Geometry: final body of the model. Coordinates: model frame, mm. Face numbers are marked on the shaded views. A direction names the side the tool comes from. Coordinates: 2 decimals unless noted, no trailing zeros. Write each loop counter-clockwise with the first axis right and the second up, starting at its lowest first coordinate (ties: lowest second). Pieces come first, ordered by that corner, then holes. Notation, with made-up numbers: M -11.75,-34 L 18.25,-34 A22 ccw 18.25,-6 Z; hole C 45.5,-10.5 d6. An arc over 180 degrees is marked long. Write item = value, one per line. Start each with the question number.
Item 1: Reachability of the marked faces 1 and 2 from +Z, -Z, +X, -X, +Y, -Y: full face, straight path, thin tool, end or side. Return the list, or none.
Item 2: First-contact query: pin 1 Ø1 at (x, y) = (10.5, -0.5) entering from -Z. Flat tip, straight axial feed; report the tip coordinate or a pass-through.
Item 3: Ray query, L1, parallel to X at y = 0.5, z = 0; L2, parallel to Y at x = -6, z = 11.5; L3, parallel to Z at x = 0.5, y = -1. Return the intervals inside material, ascending. Write a range as [from, to].
Item 4: Section D-D on y = 2.25. Output: boundary loops of the cut face in (x, z).
Item 5: Pull-direction query (Z, two-part tool) for the marked faces 3 and 4; classes: +Z half, -Z half, draft (parallel to the pull), parting line (faces both ways), or undercut.
Item 6: Section C-C on y = 7. Output: boundary loops of the cut face in (x, z), plus the area to 3 significant figures.
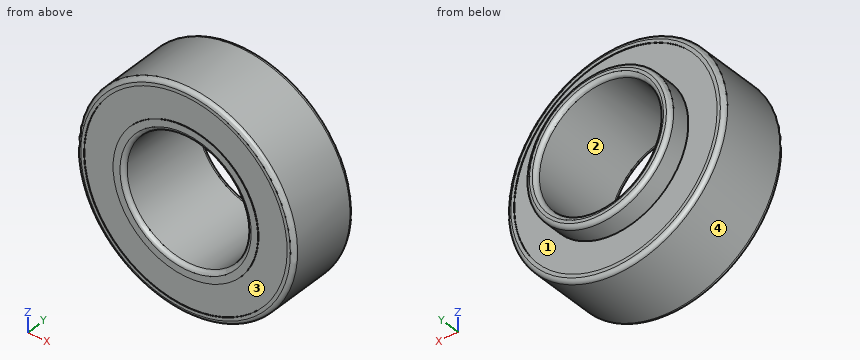
from build123d import *

# Parameters (mm, degrees)
SKETCH1_R           = 15
SKETCH1_R_2         = 8.5
BOSS_EXTRUDE1_DEPTH = 5
SKETCH2_R           = 10
SKETCH2_R_2         = 8.5
BOSS_EXTRUDE2_DEPTH = 3
CUT_EXTRUDE1_START  = -0.05
SKETCH3_R           = 14
SKETCH3_R_2         = 10
CUT_EXTRUDE1_DEPTH  = 0.05
FILLET1_R           = 0.55


with BuildPart() as part:
    # Sketch1 → Boss-Extrude1 (new, symmetric)
    with BuildSketch(Plane(origin=(0, 0, 0), x_dir=(1, 0, 0), z_dir=(0, 1, 0))):
        with Locations(Location((0, 0, 0), (0, 0, 270))):
            Circle(SKETCH1_R)
        with Locations(Location((0, 0, 0), (0, 0, 270))):
            Circle(SKETCH1_R_2, mode=Mode.SUBTRACT)
    extrude(amount=BOSS_EXTRUDE1_DEPTH, both=True)

    # Sketch2 → Boss-Extrude2 (add)
    with BuildSketch(Plane(origin=(0, 5, 0), x_dir=(1, 0, 0), z_dir=(0, 1, 0))):
        with Locations(Location((0, 0, 0), (0, 0, 270))):
            Circle(SKETCH2_R)
        with Locations(Location((0, 0, 0), (0, 0, 270))):
            Circle(SKETCH2_R_2, mode=Mode.SUBTRACT)
    extrude(amount=BOSS_EXTRUDE2_DEPTH)

    # Sketch3 → Cut-Extrude1 (cut)
    with BuildSketch(Plane(origin=(0, 5, 0), x_dir=(1, 0, 0), z_dir=(0, 1, 0)).offset(CUT_EXTRUDE1_START)):
        with Locations(Location((0, 0, 0), (0, 0, 270))):
            Circle(SKETCH3_R)
        with Locations(Location((0, 0, 0), (0, 0, 270))):
            Circle(SKETCH3_R_2, mode=Mode.SUBTRACT)
    cut_extrude1 = extrude(amount=CUT_EXTRUDE1_DEPTH, mode=Mode.SUBTRACT)

    # Mirror1: Cut-Extrude1 across plane
    add(cut_extrude1.mirror(Plane.ZX), mode=Mode.SUBTRACT)

    # Fillet1
    fillet1_edges = [part.edges().sort_by_distance(p)[0] for p in [
        (0, 8, -10),
        (0, 8, -8.5),
        (0, -5, -15),
        (0, 5, -15),
        (0, -5, -8.5),
    ]]
    fillet(fillet1_edges, radius=FILLET1_R)


solid = part.part
Responses:
q1.face_1 = +Y
q1.face_2 = +Y, -Y
q2.pin_1 = -11.18
q3.L1 = [-15, -8.5], [8.5, 15]
q3.L2 = [-4.95, 4.95]
q3.L3 = [-14.99, -8.49], [8.49, 14.99]
q4.outline = C 0,0 d30; hole C 0,0 d17
q5.face_3 = undercut
q5.face_4 = parting line
q6.outline = C 0,0 d20; hole C 0,0 d17
q6.area = 87.2 mm²
